Autodesk Inventor part; units mm, degrees
ref_plane "YZ Plane" through (0, 0, 0) normal (1, 0, 0) x (0, 1, 0)
ref_plane "XZ Plane" through (0, 0, 0) normal (0, 1, 0) x (-1, 0, 0)
ref_plane "XY Plane" through (0, 0, 0) normal (0, 0, 1) x (1, 0, 0)
sketch "Sketch1" plane through (0, 0, 0) normal (0, 1, 0) x (-1, 0, 0)
  line L0 (0, 0) -> (146, 0)
  line L1 (146, 0) -> (146, -216)
  line L2 (146, -216) -> (0, -216)
  line L3 (0, -216) -> (0, 0)
  dimension "d0" = 146
  dimension "d1" = 216
extrude "Extrusion1" add sketch "Sketch1" along normal blind 50
sketch "Sketch2" plane through (0, 50, 0) normal (0, 1, 0) x (1, 0, 0)
  point P0 (0, 0)
fillet "Fillet1" radius 37.5 2 edges at (-146, 25, 0) (0, 25, 0)
sketch "Sketch3" plane through (0, 50, 0) normal (0, 1, 0) x (1, 0, 0)
  line L0 (0, 216) -> (-146, 216)
  line L1 (-146, 216) -> (0, 216)
  line L2 (0, 216) -> (0, 37.5)
  line L3 (-37.5, 0) -> (-108.5, 0)
  line L4 (-146, 37.5) -> (-146, 216)
  arc A0 (-146, 37.5) -> (-108.5, 0) centre (-108.5, 37.5) ccw
  arc A1 (-37.5, 0) -> (0, 37.5) centre (-37.5, 37.5) ccw
  line L5 (-143, 213) -> (-3, 213)
  line L6 (-3, 213) -> (-3, 37.5)
  arc A2 (-37.5, 3) -> (-3, 37.5) centre (-37.5, 37.5) ccw
  line L7 (-37.5, 3) -> (-108.5, 3)
  arc A3 (-143, 37.5) -> (-108.5, 3) centre (-108.5, 37.5) ccw
  line L8 (-143, 37.5) -> (-143, 213)
  point P0 (0, 0)
  dimension "d5" = 37.5
  dimension "d6" = 3
extrude "Extrusion2" cut sketch "Sketch3" against normal blind 47 contours L5 L6 A2 L7 A3 L8
sketch "Sketch4" plane through (0, 3, 0) normal (0, 1, 0) x (1, 0, 0)
  circle A0 centre (-73, 60.5) radius 37.6
  circle A1 centre (-73, 155.5) radius 37.6
  line L0 (-37.5, 3) -> (-108.5, 3)
  line L1 (-3, 213) -> (-3, 37.5)
  line L2 (-143, 37.5) -> (-143, 213)
  point P0 (0, 0)
  dimension "d9" = 75.2
  dimension "d10" = 75.2
  dimension "d11" = 95
  dimension "d12" = 57.5
  dimension "d13" = 140
  dimension "d14" = 70
  dimension "d15" = 70
extrude "Extrusion3" cut sketch "Sketch4" against normal blind 47
sketch "Sketch5" plane through (0, 0, -216) normal (0, 0, -1) x (-1, 0, 0)
  line L0 (3, 50) -> (37.5, 50)
  line L1 (108.5, 3) -> (143, 3)
  line L2 (3, 50) -> (143, 50)
  line L3 (143, 50) -> (143, 3)
  line L4 (143, 3) -> (3, 3)
  line L5 (3, 3) -> (3, 50)
  point P0 (0, 0)
  point P1 (37.5, 50)
extrude "Extrusion4" cut sketch "Sketch5" against normal blind 3
sketch "Sketch6" plane through (0, 50, 0) normal (0, 1, 0) x (1, 0, 0)
  arc A0 (-143, 37.5) -> (-108.5, 3) centre (-108.5, 37.5) ccw
  line L0 (-143, 37.5) -> (-136, 37.5)
  line L1 (-136, 37.5) -> (-136, 44.5)
  line L2 (-136, 44.5) -> (-143, 44.5)
  line L3 (-143, 44.5) -> (-143, 37.5)
  line L4 (-3, 37.5) -> (-10, 37.5)
  line L5 (-10, 37.5) -> (-10, 44.5)
  line L6 (-10, 44.5) -> (-3, 44.5)
  line L7 (-3, 44.5) -> (-3, 37.5)
  line L8 (-143, 37.5) -> (-143, 216)
  line L9 (-143, 216) -> (-136, 216)
  line L10 (-136, 216) -> (-136, 209)
  line L11 (-136, 209) -> (-143, 209)
  line L12 (-143, 209) -> (-143, 216)
  line L13 (-3, 216) -> (-3, 37.5)
  line L14 (-3, 216) -> (-10, 216)
  line L15 (-10, 216) -> (-10, 209)
  line L16 (-10, 209) -> (-3, 209)
  line L17 (-3, 209) -> (-3, 216)
  point P0 (0, 0)
  point P1 (-3, 209)
  dimension "d20" = 7
  dimension "d21" = 7
  dimension "d22" = 7
  dimension "d23" = 7
  dimension "d24" = 7
  dimension "d25" = 7
  dimension "d26" = 7
  dimension "d27" = 7
extrude "Extrusion5" add sketch "Sketch6" against normal blind 50
sketch "Sketch7" plane through (0, 50, 0) normal (0, 1, 0) x (1, 0, 0)
  circle A0 centre (-139.5, 41) radius 1.45
  line L0 (-136, 44.5) -> (-143, 44.5)
  line L1 (-136, 37.5) -> (-136, 44.5)
  circle A1 centre (-139.5, 212.5) radius 1.45
  line L2 (-136, 216) -> (-146, 216)
  line L3 (-136, 209) -> (-136, 216)
  circle A2 centre (-6.5, 212.5) radius 1.45
  line L4 (-10, 216) -> (-10, 209)
  line L5 (-10, 209) -> (-3, 209)
  circle A3 centre (-6.5, 41) radius 1.45
  line L6 (-10, 44.5) -> (-10, 37.5)
  line L7 (-10, 37.5) -> (-3, 37.5)
  point P0 (0, 0)
  dimension "d34" = 2.9
  dimension "d35" = 3.5
  dimension "d36" = 3.5
  dimension "d37" = 2.9
  dimension "d38" = 3.5
  dimension "d39" = 3.5
  dimension "d40" = 2.9
  dimension "d41" = 3.5
  dimension "d42" = 3.5
  dimension "d43" = 2.9
  dimension "d44" = 3.5
  dimension "d45" = 3.5
extrude "Extrusion6" cut sketch "Sketch7" against normal blind 50
equation "\"d14\" = 0.5 * d13"
equation "\"d15\" = d14"
Source: CAD feature listing. Evaluate the final solid. Frame: model axes, mm. A direction names the side the tool comes from. Round coordinates to 2 decimals unless told otherwise and drop trailing zeros. Loops run counter-clockwise (first coordinate to the right, second up) from the corner with the lowest first, then second, coordinate; pieces in that order, holes last.
Q1. First-contact query: P1, Ø4, axis at x = -75.5, y = 42, coming from the -Z side; P2, Ø3.5, axis at x = -139.5, y = 24, coming from the +Z side; P3, Ø5.5, axis at x = -138, y = 15, coming from the +Z side. Flat tips, straight axial feed; report the tip coordinate or a pass-through.
Q2. Mould query, pull axis Z, two halves, no side actions, for faces 4 (the face through (-136, 27, -213)), 5 (the face through (-139, 27, -44.5)), 6 (the face through (-73, 25, 0)). Classes: pulls with the +Z half, pulls with the -Z half, needs draft (parallel to the pull), parting line crosses it, or undercut.
Q3. Access query for faces 1 (the face through (-7, 27, -209)), 2 (the face through (-10, 27, -213)), 3 (the face through (-73, 1, -216)). Directions: +Z, -Z, +X, -X, +Y, -Y. A direction counts if a zero-diameter tool reaches every point of the face in a straight line with its end or side. Return the directions, or none.
Q4. Section B-B, the plane y = 17. Return loops of the section in (x, z), plus the area to 3 significant figures.
Q5. Section C-C, the plane z = -60.5. Return loops of the section in (x, y), plus the area to 3 significant figures.
Q6. Ray query, line 1 (X direction, y = 14, z = -212.5); line 2 (Z direction, x = -73, y = 1); line 3 (X direction, y = 34.5, z = -173). Return the intervals inside material, ascending.
Q7. Section A-A, the plane x = -73. Return loops of the section in (y, z), plus the area to 3 significant figures.
Q8. Section D-D, the plane x = -132. Return loops of the section in (y, z).
Solutions:
1. P1: stops at z = -3
1. P2: stops at z = -14.03
1. P3: stops at z = -11.22
2. face 4: needs draft
2. face 5: undercut
2. face 6: pulls with the +Z half
3. face 1: +Y
3. face 2: -Z, +Y
3. face 3: -Z, +X, -X, +Y, -Y
4. outline: (-146, -216) - (-136, -216) - (-136, -209) - (-143, -209) - (-143, -44.5) - (-136, -44.5) - (-136, -37.5) - (-143, -37.5) arc R34.5 cw to (-108.5, -3) - (-37.5, -3) arc R34.5 cw to (-3, -37.5) - (-10, -37.5) - (-10, -44.5) - (-3, -44.5) - (-3, -209) - (-10, -209) - (-10, -216) - (0, -216) - (0, -37.5) arc R37.5 ccw to (-37.5, 0) - (-108.5, 0) arc R37.5 ccw to (-146, -37.5) - close; hole circle Ø2.9 at (-139.5, -212.5); hole circle Ø2.9 at (-139.5, -41); hole circle Ø2.9 at (-6.5, -212.5); hole circle Ø2.9 at (-6.5, -41)
4. area: 1,790 mm2
5. outline: (-146, 0) - (-110.6, 0) - (-110.6, 3) - (-143, 3) - (-143, 50) - (-146, 50) - close; (-35.4, 0) - (0, 0) - (0, 50) - (-3, 50) - (-3, 3) - (-35.4, 3) - close
5. area: 494 mm2
6. line 1: x = -146 to -140.95, -138.05 to -136, -10 to -7.95, -5.05 to 0
6. line 2: z = -216 to -193.1, -117.9 to -98.1, -22.9 to 0
6. line 3: x = -146 to -143, -3 to 0
7. outline: (0, -216) - (3, -216) - (3, -193.1) - (0, -193.1) - close; (0, -117.9) - (3, -117.9) - (3, -98.1) - (0, -98.1) - close; (0, -22.9) - (3, -22.9) - (3, -3) - (50, -3) - (50, 0) - (0, 0) - close
7. area: 338 mm2
8. outline: (0, -216) - (3, -216) - (3, -12.24) - (50, -12.24) - (50, -8.28) - (0, -8.28) - close
